Here's how the part is built. I have some questions about the finished solid (model axes, mm). A direction names the side the tool comes from. Round coordinates to 2 decimals unless told otherwise and drop trailing zeros. Write each loop counter-clockwise with the first axis right and the second up, starting at its lowest first coordinate (ties: lowest second). Pieces come first, ordered by that corner, then holes. Notation, with made-up numbers: M 89.5,-14.75 L 133.5,-14.75 A27 cw 133.5,24.25 Z; hole C 80.5,32.5 d9. An arc over 180 degrees is marked long. Use one line per item in the form item = value. Start each with the question number.
Q1. I'm going to push flat-ended pins straight in: pin 1 Ø5 at (x, z) = (4, 4) entering from -Y; pin 2 Ø3 at (y, z) = (-5, 24) entering from +X; pin 3 Ø10 at (y, z) = (-19.5, 24.5) entering from +X. Where does each tip first touch, or does it pass through?
Q2. I want a section at D-D on x = 42.5. List the corners of the cut face in (y, z) for me, and give its area (3 significant figures).
Q3. I want a section at A-A on y = -6.5. List the corners of the cut face in (x, z) for me.
Q4. I need wall thicknesses on line 1 along Z through (x, y) = (51, -7.5); line 2 along Y through (x, z) = (42.5, 41); line 3 along Z through (x, y) = (24, -11.5). Which ranges of each line are inside material? Lowest first, please. Write a range as from..to.
Q5. I want a section at B-B on z = 24. List the corners of the cut face in (x, y) for me, and give its area (3 significant figures).
Q6. For faces 1 (the face through (10, -18, 21)), 2 (the face through (5, -20, 8)), 3 (the face through (40, -20, 40)), 4 (the face through (53, -5, 15)), which set-ups out of +Z, -Z, +X, -X, +Y, -Y let a thin tool reach every point of the face, with its end or its side?
Q7. I want a section at C-C on x = 5. List the corners of the cut face in (y, z) for me.
```python
from build123d import *

# Parameters (mm, degrees)
F1_DEPTH = 30
F2_DEPTH = 10
F0_W     = 10
F0_H     = 15
F3_DEPTH = 20


with BuildPart() as f1:
    # F0 (on Front) → F1 (new body)
    with BuildSketch(Plane.XZ):
        Polygon((0, 45), (0, 15), (10, 15), (10, 35), (40, 35), (40, 45), align=None)
    extrude(amount=F1_DEPTH)

    # F0 (on Front) → F2 (join)
    with BuildSketch(Plane.XZ):
        Polygon((10, 15), (10, 0), (60, 0), (60, 15), (45, 15), (45, 30), (60, 30), (60, 45), (40, 45), (40, 35), (10, 35), align=None)
    extrude(amount=F2_DEPTH)

    # F0 (on Front) → F3 (join)
    with BuildSketch(Plane.XZ):
        with Locations((5, 7.5)):
            Rectangle(F0_W, F0_H)
    extrude(amount=F3_DEPTH)


solid = f1.part
```
Reported:
q1.pin_1 = -20
q1.pin_2 = 45
q1.pin_3 = 10
q2.outline = M -10,0 L 0,0 L 0,45 L -10,45 Z
q2.area = 450 mm^2
q3.outline = M 0,0 L 60,0 L 60,15 L 45,15 L 45,30 L 60,30 L 60,45 L 0,45 Z
q4.line_1 = 0..15, 30..45
q4.line_2 = -10..0
q4.line_3 = 35..45
q5.outline = M 0,-30 L 10,-30 L 10,-10 L 45,-10 L 45,0 L 0,0 Z
q5.area = 650 mm^2
q6.face_1 = -Z, +X, -Y
q6.face_2 = -Z, +X, -X, -Y
q6.face_3 = +Z, -Z, +X, -Y
q6.face_4 = +X, +Y, -Y
q7.outline = M -30,15 L -20,15 L -20,0 L 0,0 L 0,45 L -30,45 Z
